Work out the finished part from the listing and answer in its coordinate system (mm). A direction names the side the tool comes from. Round coordinates to 2 decimals unless told otherwise and drop trailing zeros. Loops run counter-clockwise (first coordinate to the right, second up) from the corner with the lowest first, then second, coordinate; pieces in that order, holes last. Notation, with made-up numbers: (61.5, 59) - (110.5, 59) arc R12 cw to (110.5, 73) - close; hole circle Ø1 at (88, 38). An arc over 180 degrees is marked (long way). Answer as CSV lines item,"result". Start each with the question number.
Q1. Straight lines are drawn through the part: L1, parallel to Z at x = 3.25, y = 5; L2, parallel to X at y = 3.75, z = 4; L3, parallel to Y at x = 5.75, z = 3.5. For each, find the intervals that lie inside material, in ascending order. Write a range as [from, to].
Q2. Each of these flat-tipped pins is pushed along its axis until it touches: pin 1 Ø0.9 at (y, z) = (3, -0.5) entering from -X; pin 2 Ø0.6 at (y, z) = (4, -0.5) entering from +X; pin 3 Ø2 at (x, y) = (12.5, 5) entering from -Z. Where does it stop, or does it pass through?
Q3. For faces 1 (the face through (11.479, 3.9, -0.5)), 2 (the face through (9, 0, 2)), 3 (the face through (12.479, 3.9, -0.5)), determine the directions among +Z, -Z, +X, -X, +Y, -Y from which every point of the face is accessible in a straight line to the end or side of a thin tool.
Q4. Section A-A on y = 2.75 is taken. Write down the section's boundary in (x, z), then the cut area to 3 significant figures.
Q5. Section C-C on y = 7 is taken. Write down the section's boundary in (x, z), then the cut area to 3 significant figures.
```python
from build123d import *
from build123d.topology import SkipClean

# Parameters (mm, degrees)
ESQUISSE1_W                  = 18
ESQUISSE1_H                  = 7.75
BOSS_EXTRU_1_DEPTH           = 5
ENL_V_MAT_EXTRU_1_DEPTH      = 15
ENL_V_MAT_EXTRU_1_DEPTH_BACK = 10
ESQUISSE13_RX                = 0.8
ESQUISSE13_RY                = 0.6
ESQUISSE15_R                 = 0.5
BOSS_EXTRU_3_DEPTH           = 0.55
BOSS_EXTRU_4_DEPTH           = 1.1


with BuildPart() as part:
    # Esquisse1 → Boss.-Extru.1 (new body)
    with BuildSketch(Plane.XY):
        with Locations((9, 3.875)):
            Rectangle(ESQUISSE1_W, ESQUISSE1_H)
    extrude(amount=BOSS_EXTRU_1_DEPTH)

    # Esquisse13 → Enl_v. mat.-Extru.1 (cut, two sides: drawn at the far end of the back side and taken through both)
    with BuildSketch(Plane(origin=(5, 3.875, 5), x_dir=(-0.7071067811865476, 0, -0.7071067811865475), z_dir=(0.7071067811865475, 0, -0.7071067811865476)).offset(-ENL_V_MAT_EXTRU_1_DEPTH_BACK)):
        with Locations(Location((0, 0), (0, 0, 0))):
            Ellipse(ESQUISSE13_RX, ESQUISSE13_RY)
    extrude(amount=ENL_V_MAT_EXTRU_1_DEPTH + ENL_V_MAT_EXTRU_1_DEPTH_BACK, mode=Mode.SUBTRACT)

    # Esquisse15 → Boss.-Extru.3 (add)
    with BuildSketch(Plane(origin=(0, 0, 0), x_dir=(-1, 0, 0), z_dir=(0, 0, -1))):
        with Locations(Location((-11.979236125, 2.375, 0), (0, 0, 180))):
            Circle(ESQUISSE15_R)
        with Locations(Location((-11.979236125, 5.375, 0), (0, 0, 180))):
            Circle(ESQUISSE15_R)
    extrude(amount=BOSS_EXTRU_3_DEPTH)

    # Esquisse16 → Boss.-Extru.4 (add)
    with SkipClean():  # the faces are left unmerged after this step: merging them gives an invalid solid
        with BuildSketch(Plane(origin=(0, 0, 0), x_dir=(-1, 0, 0), z_dir=(0, 0, -1))):
            with BuildLine():
                Line((-12.479236125, 2.375), (-12.479236125, 5.375))
                ThreePointArc((-12.479236125, 5.375), (-11.979236125, 5.875), (-11.479236125, 5.375))
                Line((-11.479236125, 5.375), (-11.479236125, 2.375))
                ThreePointArc((-11.479236125, 2.375), (-11.979236125, 1.875), (-12.479236125, 2.375))
            make_face()
        extrude(amount=BOSS_EXTRU_4_DEPTH)


solid = part.part
```
Findings:
1,L1,"z = [0, 5]"
1,L2,"x = [0, 4.89], [7.11, 18]"
1,L3,"y = [0, 3.43], [4.32, 7.75]"
2,pin 1,"stops at x = 11.48"
2,pin 2,"stops at x = 12.48"
2,pin 3,"stops at z = -1.1"
3,face 1,"-Z, -X, +Y, -Y"
3,face 2,"+Z, -Z, +X, -X, -Y"
3,face 3,"-Z, +X, +Y, -Y"
4,outline,"(0, 0) - (11.48, 0) - (11.48, -1.1) - (12.48, -1.1) - (12.48, 0) - (18, 0) - (18, 5) - (0, 5) - close"
4,area,"91.1 mm^2"
5,outline,"(0, 0) - (18, 0) - (18, 5) - (0, 5) - close"
5,area,"90.0 mm^2"
